```python
from build123d import *

# Parameters (mm, degrees)
BOSS_EXTRUDE1_DEPTH = 5
CUT_EXTRUDE1_DEPTH  = 2
CUT_EXTRUDE2_DEPTH  = 1
CUT_EXTRUDE3_DEPTH  = 71.887234394
SKETCH5_R           = 9
CUT_EXTRUDE4_DEPTH  = 1
SKETCH6_R           = 1.5
CUT_EXTRUDE5_DEPTH  = 71.823724839


with BuildPart() as part:
    # Sketch1 → Boss-Extrude1 (new body)
    with BuildSketch(Plane(origin=(0, 0, 0), x_dir=(1, 0, 0), z_dir=(0, 1, 0))):
        with BuildLine():
            Line((-50, 10), (-60, 10))
            ThreePointArc((-60, 10), (-70, 0), (-60, -10))
            Line((-60, -10), (50, -10))
            ThreePointArc((50, -10), (60, 0), (50, 10))
            Line((50, 10), (-50, 10))
        make_face()
    extrude(amount=BOSS_EXTRUDE1_DEPTH)

    # Sketch2 → Cut-Extrude1 (cut)
    with BuildSketch(Plane.XZ):
        with BuildLine():
            ThreePointArc((50, 4), (46, 0), (50, -4))
            Line((50, -4), (50, 4))
        make_face()
        with BuildLine():
            Line((50, 4), (50, -4))
            ThreePointArc((50, -4), (52.828427125, -2.828427125), (54, 0))
            ThreePointArc((54, 0), (52.828427125, 2.828427125), (50, 4))
        make_face()
    extrude(amount=-CUT_EXTRUDE1_DEPTH, mode=Mode.SUBTRACT)

    # Sketch3 → Cut-Extrude2 (cut)
    with BuildSketch(Plane(origin=(0, 5, 0), x_dir=(1, 0, 0), z_dir=(0, 1, 0))):
        with BuildLine():
            ThreePointArc((53, 0), (52.121320344, 2.121320344), (50, 3))
            Line((50, 3), (50, -3))
            ThreePointArc((50, -3), (52.121320344, -2.121320344), (53, 0))
        make_face()
        with BuildLine():
            Line((50, -3), (50, 3))
            ThreePointArc((50, 3), (47, 0), (50, -3))
        make_face()
    extrude(amount=-CUT_EXTRUDE2_DEPTH, mode=Mode.SUBTRACT)

    # Sketch4 → Cut-Extrude3 (cut, through all)
    with BuildSketch(Plane(origin=(0, 5, 0), x_dir=(1, 0, 0), z_dir=(0, 1, 0))):
        with BuildLine():
            ThreePointArc((-52, 0), (-54.343145751, 5.656854249), (-60, 8))
            Line((-60, 8), (-60, -8))
            ThreePointArc((-60, -8), (-54.343145751, -5.656854249), (-52, 0))
        make_face()
        with BuildLine():
            Line((-60, -8), (-60, 8))
            ThreePointArc((-60, 8), (-68, 0), (-60, -8))
        make_face()
    extrude(amount=-CUT_EXTRUDE3_DEPTH, mode=Mode.SUBTRACT)

    # Sketch5 → Cut-Extrude4 (cut)
    with BuildSketch(Plane(origin=(0, 5, 0), x_dir=(1, 0, 0), z_dir=(0, 1, 0))):
        with Locations(Location((-60, 0, 0), (0, 0, 270))):
            Circle(SKETCH5_R)
    extrude(amount=-CUT_EXTRUDE4_DEPTH, mode=Mode.SUBTRACT)

    # Sketch6 → Cut-Extrude5 (cut, through all)
    with BuildSketch(Plane(origin=(0, 4, 0), x_dir=(1, 0, 0), z_dir=(0, 1, 0))):
        with Locations(Location((50, 0, 0), (0, 0, 270))):
            Circle(SKETCH6_R)
    extrude(amount=-CUT_EXTRUDE5_DEPTH, mode=Mode.SUBTRACT)


solid = part.part
```
Work out the finished part from the listing and answer in its coordinate system (mm). A direction names the side the tool comes from. Coordinates: 2 decimals unless noted, no trailing zeros. Loops run counter-clockwise (first coordinate to the right, second up) from the corner with the lowest first, then second, coordinate; pieces in that order, holes last.
1) For a pull along Z with two mould halves and no side action, classify faces 1 (the cylindrical face through (-68.786, 4.507, -1.951)), 2 (the flat face through (-4, 2, -10)), 3 (the cylindrical face through (60, 2, 0)) as +Z half, -Z half, draft (parallel to the pull), parting line (faces both ways), or undercut.
Results:
face 1: undercut
face 2: -Z half
face 3: parting line
2) For faces 4 (the flat face through (50, 2, -2)), 5 (the flat face through (51.3, 4, 1.3)), 6 (the flat face through (-6, 0, 0)), determine the directions among +Z, -Z, +X, -X, +Y, -Y from which every point of the face is accessible in a straight line to the end or side of a thin tool.
Results:
face 4: -Y
face 5: +Y
face 6: +Z, -Z, +X, -X, -Y
3) Section A-A (z = 6) is taken. Give the vertices of the cut face in (x, y), plus the area to 3 significant figures.
Results:
outline: (-68, 0) - (-65.29, 0) - (-65.29, 4) - (-66.71, 4) - (-66.71, 5) - (-68, 5) - close; (-54.71, 0) - (58, 0) - (58, 5) - (-53.29, 5) - (-53.29, 4) - (-54.71, 4) - close
area: 574 mm2
4) Flat-ended cylindrical pins translate along their axes: pin 1 (12 mm diameter, centred on x = -27, z = -5.5, fed in from -Y); pin 2 (2.5 mm diameter, centred on x = 49, z = 1, fed in from -Y); pin 3 (3 mm diameter, centred on x = 50, z = 1, fed in from +Y); pin 4 (1 mm diameter, centred on y = 3, z = -5.5, fed in from -X). Find the tip coordinate at first contact, or state that the pin passes through.
Results:
pin 1: stops at y = 0
pin 2: stops at y = 2
pin 3: stops at y = 4
pin 4: stops at x = -68.66
5) Section B-B (y = 3) is taken. Give the vertices of the cut face in (x, z).
Results:
outline: (-60, -10) - (50, -10) arc R10 ccw to (50, 10) - (-60, 10) arc R10 ccw to start; hole circle Ø16 at (-60, 0); hole circle Ø3 at (50, 0)
6) Consider probe 1 along X at (y, z) = (1.65, 0.25); probe 2 along X at (y, z) = (4.55, 0); probe 3 along X at (y, z) = (4.3, -4.5). Determine where each line is inside the solid, lowest interval first.
Results:
probe 1: x = -70 to -68, -52 to 46.01, 53.99 to 60
probe 2: x = -70 to -69, -51 to 47, 53 to 60
probe 3: x = -68.93 to -67.79, -52.21 to 58.93
